from build123d import *

# Parameters (mm, degrees)
SKETCH1_R           = 6.3
BOSS_EXTRUDE1_DEPTH = 6
SKETCH2_R           = 1.25
BOSS_EXTRUDE2_DEPTH = 0.9
SKETCH3_R           = 0.5
BOSS_EXTRUDE3_DEPTH = 3.5


with BuildPart() as part:
    # Sketch1 → Boss-Extrude1 (new body)
    with BuildSketch(Plane(origin=(0, 0, 0), x_dir=(1, 0, 0), z_dir=(0, 1, 0))):
        with Locations(Location((0, 0, 0), (0, 0, 270))):
            Circle(SKETCH1_R)
    extrude(amount=BOSS_EXTRUDE1_DEPTH)

    # Sketch2 → Boss-Extrude2 (add)
    with BuildSketch(Plane.XZ):
        with Locations(Location((2.5, 0, 0), (0, 0, 90))):
            Circle(SKETCH2_R)
    boss_extrude2 = extrude(amount=BOSS_EXTRUDE2_DEPTH)

    # Sketch3 → Boss-Extrude3 (add)
    with BuildSketch(Plane.XZ.offset(0.9)):
        with Locations(Location((2.5, 0, 0), (0, 0, 270))):
            Circle(SKETCH3_R)
    boss_extrude3 = extrude(amount=BOSS_EXTRUDE3_DEPTH)

    # Mirror1: Boss-Extrude2, Boss-Extrude3 across plane
    add(boss_extrude2.mirror(Plane(origin=(0, 0, 0), x_dir=(0, 0, 1), z_dir=(1, 0, 0))))
    add(boss_extrude3.mirror(Plane(origin=(0, 0, 0), x_dir=(0, 0, 1), z_dir=(1, 0, 0))))


solid = part.part
The model under review builds one solid part; all positions refer to its coordinate system, in mm. A direction names the side the tool comes from. Coordinates: 2 decimals unless noted, no trailing zeros. Loops run counter-clockwise (first coordinate to the right, second up) from the corner with the lowest first, then second, coordinate; pieces in that order, holes last. Notation, with made-up numbers: (-2, 56) -> (49, 56) arc R33 cw to (49, 95) -> close; hole circle Ø10 at (72.25, 22.25). An arc over 180 degrees is marked (long way). Use a Markdown table: item, result. Add a question column.
1. Machinability: for faces 1 (the face through (3, -3, 0)), 2 (the face through (-3.83, 2.96, -5)), which of the approach directions +Z, -Z, +X, -X, +Y, -Y give a long, thin tool a straight path to every point of the face, cutting with its end or side? Answer none if there is none.
2. To check wall thickness, follow line 1 (Y direction, x = -0.5, z = 3.5); line 2 (Z direction, x = -2.5, y = -3.75); line 3 (X direction, y = 1.75, z = 5.25). State the ranges of each line that lie inside material, in increasing order.
3. Add section A-A on z = 0. Write out the cut boundary in (x, y), plus the area to 3 significant figures.
4. Add section B-B on y = -0.5. Write out the cut boundary in (x, z).
5. Clearance check with flat-ended pins moving along their axes: pin 1 Ø1 at (x, y) = (-3, 1) entering from -Z; pin 2 Ø2 at (x, z) = (-4, 0.5) entering from -Y; pin 3 Ø3 at (y, z) = (-2, 4) entering from -X. State where each tip first meets the part, or that it passes through.
6. Add section D-D on y = 1.5. Write out the cut boundary in (x, z), plus the area to 3 significant figures.
7. Add section C-C on x = 1.75. Write out the cut boundary in (y, z), plus the area to 3 significant figures.
Returned:
| question | item | result |
|---|---|---|
| 1 | face 1 | -Y |
| 1 | face 2 | +Y, -Y |
| 2 | line 1 | y = 0 to 6 |
| 2 | line 2 | z = -0.5 to 0.5 |
| 2 | line 3 | x = -3.48 to 3.48 |
| 3 | outline | (-6.3, 0) -> (-3.75, 0) -> (-3.75, -0.9) -> (-3, -0.9) -> (-3, -4.4) -> (-2, -4.4) -> (-2, -0.9) -> (-1.25, -0.9) -> (-1.25, 0) -> (1.25, 0) -> (1.25, -0.9) -> (2, -0.9) -> (2, -4.4) -> (3, -4.4) -> (3, -0.9) -> (3.75, -0.9) -> (3.75, 0) -> (6.3, 0) -> (6.3, 6) -> (-6.3, 6) -> close |
| 3 | area | 87.1 mm² |
| 4 | outline | circle Ø2.5 at (-2.5, 0); circle Ø2.5 at (2.5, 0) |
| 5 | pin 1 | stops at z = -5.78 |
| 5 | pin 2 | stops at y = -0.9 |
| 5 | pin 3 | passes through |
| 6 | outline | circle Ø12.6 at (0, 0) |
| 6 | area | 125 mm² |
| 7 | outline | (-0.9, -1) -> (0, -1) -> (0, -6.05) -> (6, -6.05) -> (6, 6.05) -> (0, 6.05) -> (0, 1) -> (-0.9, 1) -> close |
| 7 | area | 74.4 mm² |
